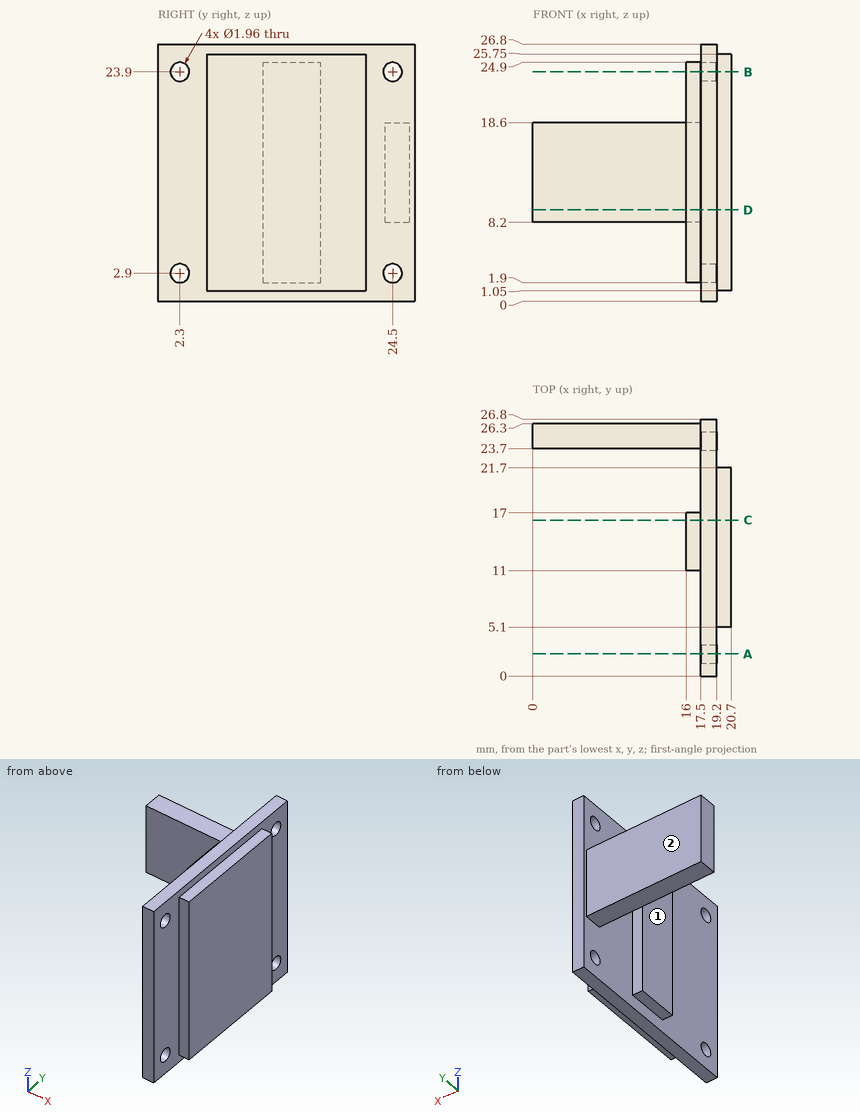
Drawing for the job (mm, zero at the part's lowest x, y, z). Round coordinates to 2 decimals unless told otherwise and drop trailing zeros. Loops run counter-clockwise (first coordinate to the right, second up) from the corner with the lowest first, then second, coordinate; pieces in that order, holes last. Notation, with made-up numbers: M 0.25,34 L 59.25,34 A23 ccw 59.25,69 Z; hole C 59,10 d11. An arc over 180 degrees is marked long. Use a Markdown table: item, result. Add a question column.
(1) Cut at D-D (z = 9.5). Give the cut face in (x, y), and give its area (3 significant figures).
(2) Cut at B-B (z = 23.9). Give the cut face in (x, y).
(3) Cut at A-A (y = 2.3). Give the cut face in (x, z), and give its area (3 significant figures).
(4) Pull direction Y, two halves, no side cores. Call the marked faces 1 and 2: +Y half, -Y half, draft (parallel to the pull), parting line (faces both ways), or undercut.
(5) Cut at C-C (y = 16.25). Give the cut face in (x, z), and give its area (3 significant figures).
(6) Flat gauge pins, fed straight in: pin 1 (1.6 mm diameter, centred on x = 16.5, y = 15, fed in from -Z); pin 2 (1.2 mm diameter, centred on x = 20, y = 11.5, fed in from +Z); pin 3 (3 mm diameter, centred on y = 24.5, z = 2.9, fed in from +X); pin 4 (12 mm diameter, centred on y = 21.5, z = 16, fed in from -X). Where does each tip first touch, or does it go through?
(7) Drill centre lines: line 1 (Y direction, x = 18.7, z = 23.9); line 2 (Y direction, x = 4, z = 11.5); line 3 (X direction, y = 19.5, z = 23.25). Where is each one in solid material? Low to high.
Geometry says:
| question | item | result |
|---|---|---|
| 1 | outline | M 0,23.7 L 17.5,23.7 L 17.5,17 L 16,17 L 16,11 L 17.5,11 L 17.5,0 L 19.2,0 L 19.2,5.1 L 20.7,5.1 L 20.7,21.7 L 19.2,21.7 L 19.2,26.8 L 17.5,26.8 L 17.5,26.3 L 0,26.3 Z |
| 1 | area | 125 mm² |
| 2 | outline | M 16,11 L 17.5,11 L 17.5,3.28 L 19.2,3.28 L 19.2,5.1 L 20.7,5.1 L 20.7,21.7 L 19.2,21.7 L 19.2,23.52 L 17.5,23.52 L 17.5,17 L 16,17 Z; M 17.5,0 L 19.2,0 L 19.2,1.32 L 17.5,1.32 Z; M 17.5,25.48 L 19.2,25.48 L 19.2,26.8 L 17.5,26.8 Z |
| 3 | outline | M 17.5,0 L 19.2,0 L 19.2,1.92 L 17.5,1.92 Z; M 17.5,3.88 L 19.2,3.88 L 19.2,22.92 L 17.5,22.92 Z; M 17.5,24.88 L 19.2,24.88 L 19.2,26.8 L 17.5,26.8 Z |
| 3 | area | 38.9 mm² |
| 4 | face 1 | draft |
| 4 | face 2 | +Y half |
| 5 | outline | M 16,1.9 L 17.5,1.9 L 17.5,0 L 19.2,0 L 19.2,1.05 L 20.7,1.05 L 20.7,25.75 L 19.2,25.75 L 19.2,26.8 L 17.5,26.8 L 17.5,24.9 L 16,24.9 Z |
| 5 | area | 117 mm² |
| 6 | pin 1 | stops at z = 1.9 |
| 6 | pin 2 | stops at z = 25.75 |
| 6 | pin 3 | stops at x = 19.2 |
| 6 | pin 4 | stops at x = 0 |
| 7 | line 1 | y = 0 to 1.32, 3.28 to 23.52, 25.48 to 26.8 |
| 7 | line 2 | y = 23.7 to 26.3 |
| 7 | line 3 | x = 17.5 to 20.7 |
